Can you work these out from the model? Positions are in its coordinate system, mm. A direction names the side the tool comes from. Coordinates: 2 decimals unless noted, no trailing zeros. Order: outer loops, then holes, each group sorted by start corner. A loop starts at its lowest first (then second) coordinate and runs counter-clockwise, first axis right, second up. Notation, with made-up numbers: (75.5, 1.25) - (111.5, 1.25) arc R15 ccw to (111.5, 5.25) - close; hole circle Ø8 at (78, -8). An arc over 180 degrees is marked (long way). Return JSON: item names as keys, results as strings. Group by question number.
1) If I drill on line 1 along Z through (x, y) = (-7.5, -1.05); line 2 along Z through (x, y) = (-16, -1.2); line 3 along X through (y, z) = (-2.25, 7.5), over which ranges is the centre line in solid material (lowest first)?
2) Imagine slicing it at C-C (x = 13). Write out the boundary of the cut face in (y, z), and give its area (3 significant figures).
3) Imagine slicing it at A-A (z = -7.5). Write out the boundary of the cut face in (x, y).
4) Imagine slicing it at D-D (y = -0.7). Write out the boundary of the cut face in (x, z).
5) Imagine slicing it at B-B (x = -15.5). Write out the boundary of the cut face in (y, z).
6) If we mould it in two halves opening along Z, with no side actions, what happens to faces 4 (the face through (0, -1, -15)), 5 (the face through (4, -1, 4)), 6 (the face through (-19.1, -1.48, 14.14))? For each: pulls with the +Z half, pulls with the -Z half, needs draft (parallel to the pull), parting line crosses it, or undercut.
7) Which directions (+Z, -Z, +X, -X, +Y, -Y) give clear straight access to the entire face, cutting with the end or side of a thin tool? Please do faces 1 (the face through (-13.9, -1.48, -9.43)), 2 (the face through (-19.14, -1.48, -14.1)), 3 (the face through (-13.9, -1.48, 4.57)).
```python
from build123d import *

# Parameters (mm, degrees)
F1_DEPTH = 3


with BuildPart() as f1:
    # F0 (on Front) → F1 (new body)
    with BuildSketch(Plane.XZ):
        with BuildLine():
            ThreePointArc((20, 12), (19.12132, 14.12132), (17, 15))
            Line((17, 15), (-17, 15))
            ThreePointArc((-17, 15), (-19.12132, 14.12132), (-20, 12))
            Line((-20, 12), (-20, -4))
            Line((-20, -4), (12.5, -4))
            ThreePointArc((12.5, -4), (13.914214, -4.585786), (14.5, -6))
            Line((14.5, -6), (14.5, -8))
            ThreePointArc((14.5, -8), (13.914214, -9.414214), (12.5, -10))
            Line((12.5, -10), (-12.5, -10))
            ThreePointArc((-12.5, -10), (-13.914214, -9.414214), (-14.5, -8))
            Line((-14.5, -8), (-14.5, -7))
            Line((-14.5, -7), (-20, -7))
            Line((-20, -7), (-20, -12))
            ThreePointArc((-20, -12), (-19.12132, -14.12132), (-17, -15))
            Line((-17, -15), (17, -15))
            ThreePointArc((17, -15), (19.12132, -14.12132), (20, -12))
            Line((20, -12), (20, 4))
            Line((20, 4), (-12.5, 4))
            ThreePointArc((-12.5, 4), (-13.914214, 4.585786), (-14.5, 6))
            Line((-14.5, 6), (-14.5, 8))
            ThreePointArc((-14.5, 8), (-13.914214, 9.414214), (-12.5, 10))
            Line((-12.5, 10), (12.5, 10))
            ThreePointArc((12.5, 10), (13.914214, 9.414214), (14.5, 8))
            Line((14.5, 8), (14.5, 7))
            Line((14.5, 7), (20, 7))
            Line((20, 7), (20, 12))
        make_face()
    extrude(amount=F1_DEPTH)


solid = f1.part
```
Calculated:
{
 "1": {"line 1": "-15 to -10, -4 to 4, 10 to 15", "line 2": "-15 to -7, -4 to 15", "line 3": "-20 to -14.5, 14.5 to 20"},
 "2": {"outline": "(-3, -15) - (0, -15) - (0, -9.94) - (-3, -9.94) - close; (-3, -4.06) - (0, -4.06) - (0, 4) - (-3, 4) - close; (-3, 9.94) - (0, 9.94) - (0, 15) - (-3, 15) - close", "area": "54.6 mm2"},
 "3": {"outline": "(-20, -3) - (-14.5, -3) - (-14.5, 0) - (-20, 0) - close; (14.5, -3) - (20, -3) - (20, 0) - (14.5, 0) - close"},
 "4": {"outline": "(-20, -12) arc R3 ccw to (-17, -15) - (17, -15) arc R3 ccw to (20, -12) - (20, 4) - (-12.5, 4) arc R2 cw to (-14.5, 6) - (-14.5, 8) arc R2 cw to (-12.5, 10) - (12.5, 10) arc R2 cw to (14.5, 8) - (14.5, 7) - (20, 7) - (20, 12) arc R3 ccw to (17, 15) - (-17, 15) arc R3 ccw to (-20, 12) - (-20, -4) - (12.5, -4) arc R2 cw to (14.5, -6) - (14.5, -8) arc R2 cw to (12.5, -10) - (-12.5, -10) arc R2 cw to (-14.5, -8) - (-14.5, -7) - (-20, -7) - close"},
 "5": {"outline": "(-3, -15) - (0, -15) - (0, -7) - (-3, -7) - close; (-3, -4) - (0, -4) - (0, 15) - (-3, 15) - close"},
 "6": {"face 4": "pulls with the -Z half", "face 5": "undercut", "face 6": "pulls with the +Z half"},
 "7": {"face 1": "+Y, -Y", "face 2": "-Z, -X, +Y, -Y", "face 3": "+X, +Y, -Y"}
}
